Check sheet for the drawn part. Datum: minimum x, y, z corner. Units: mm. Round coordinates to 2 decimals unless told otherwise and drop trailing zeros. Write each loop counter-clockwise with the first axis right and the second up, starting at its lowest first coordinate (ties: lowest second). Pieces come first, ordered by that corner, then holes. Notation, with made-up numbers: (-4.5, -28.75) - (1.5, -28.75) arc R31 cw to (1.5, 6.25) - close; hole circle Ø7 at (-4.75, 39). An arc over 180 degrees is marked (long way). Answer as a JSON object with one key per item and string values. Group by question number.
Item 1: Release check for a two-part mould opening along Y. For the marked faces 1, 2 and 3 record: pulls with the +Y half, pulls with the -Y half, needs draft (parallel to the pull), parting line crosses it, or undercut.
Item 2: Thickness scan on line 1 (Y direction, x = 3.5, z = 3.5); line 2 (Y direction, x = 4.5, z = 0.75); line 3 (X direction, y = 2, z = 7.75). Record the ranges inside material, lowest first.
Item 3: Sectioned sample at A-A on x = 3.5. Record the boundary of the cut face in (y, z).
Item 4: Sectioned sample at B-B on z = 8.75. Record the boundary of the cut face in (x, y).
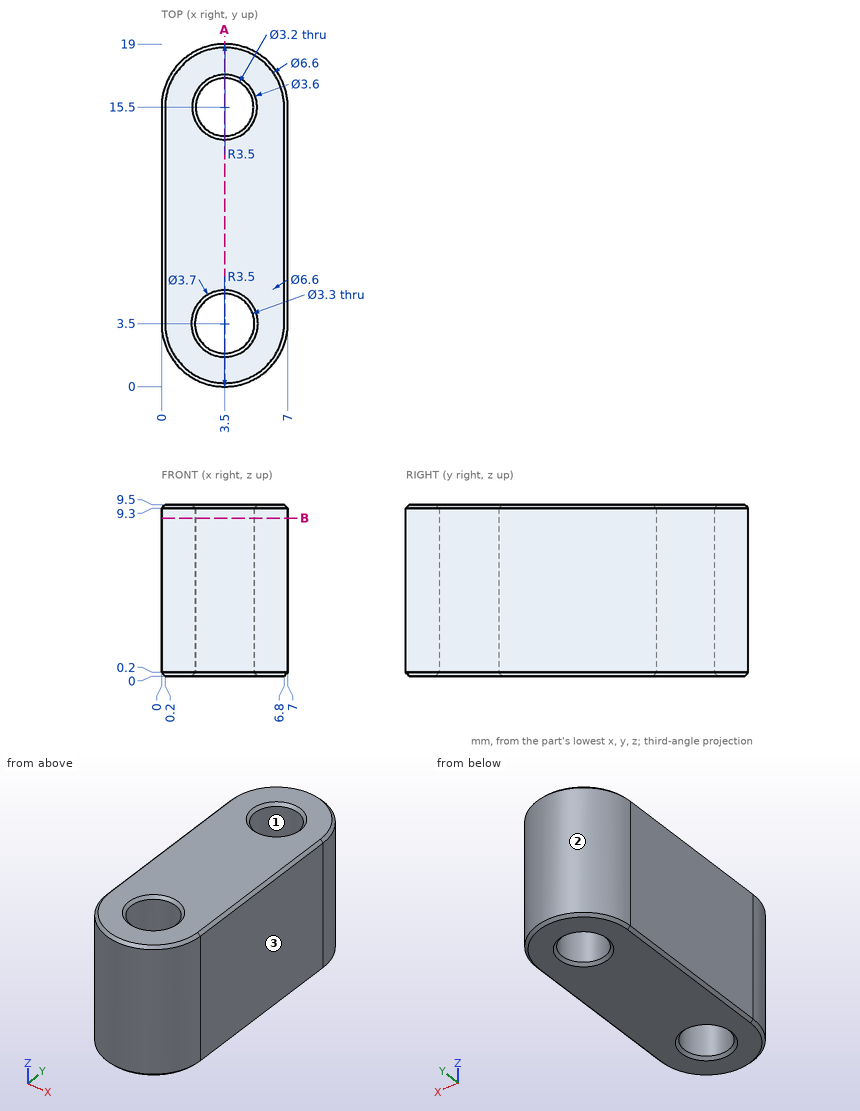
Completed:
{
 "1": {"face 1": "undercut", "face 2": "pulls with the +Y half", "face 3": "needs draft"},
 "2": {"line 1": "0 to 1.85, 5.15 to 13.9, 17.1 to 19", "line 2": "0.15 to 2.19, 4.81 to 14.25, 16.75 to 18.85", "line 3": "0.34 to 2.81, 4.19 to 6.66"},
 "3": {"outline": "(0, 0.2) - (0.2, 0) - (1.65, 0) - (1.85, 0.2) - (1.85, 9.3) - (1.65, 9.5) - (0.2, 9.5) - (0, 9.3) - close; (5.15, 0.2) - (5.35, 0) - (13.7, 0) - (13.9, 0.2) - (13.9, 9.3) - (13.7, 9.5) - (5.35, 9.5) - (5.15, 9.3) - close; (17.1, 0.2) - (17.3, 0) - (18.8, 0) - (19, 0.2) - (19, 9.3) - (18.8, 9.5) - (17.3, 9.5) - (17.1, 9.3) - close"},
 "4": {"outline": "(0, 3.5) arc R3.5 ccw to (7, 3.5) - (7, 15.5) arc R3.5 ccw to (0, 15.5) - close; hole circle Ø3.3 at (3.5, 3.5); hole circle Ø3.2 at (3.5, 15.5)"}
}
